Autodesk Inventor part; units mm, degrees
ref_plane "YZ Plane" through (0, 0, 0) normal (1, 0, 0) x (0, 1, 0)
ref_plane "XZ Plane" through (0, 0, 0) normal (0, 1, 0) x (-1, 0, 0)
ref_plane "XY Plane" through (0, 0, 0) normal (0, 0, 1) x (1, 0, 0)
sketch "Sketch1" plane through (0, 0, 0) normal (0, 1, 0) x (-1, 0, 0)
  line L0 (0, 0) -> (90, 0)
  line L1 (90, 0) -> (90, -45)
  line L2 (90, -45) -> (0, -45)
  line L3 (0, -45) -> (0, 0)
  dimension "d0" = 90
  dimension "d1" = 45
extrude "Extrusion1" add sketch "Sketch1" along normal blind 45
sketch "Sketch2" plane through (0, 45, 0) normal (0, 1, 0) x (1, 0, 0)
  point P0 (0, 0)
shell "Shell1" thickness 1.5 removed faces 1 at (-30, 45, -15)
sketch "Sketch3" plane through (-90, 0, 0) normal (0, 0, 1) x (1, 0, 0)
  line L0 (75, 35) -> (65, 35)
  line L1 (1.5, 45) -> (88.5, 45)
  line L2 (75, 35) -> (65, 35)
  line L3 (65, 35) -> (65, 45)
  line L4 (65, 45) -> (75, 45)
  line L5 (75, 45) -> (75, 35)
  point P0 (90, 0)
extrude "Extrusion2" cut sketch "Sketch3" against normal blind 10
sketch "Sketch4" plane through (0, 0, -45) normal (0, 0, -1) x (-1, 0, 0)
  line L0 (45, 45) -> (53.3446, 45)
  line L1 (53.3446, 45) -> (53.3446, 39.0799)
  line L2 (53.3446, 39.0799) -> (45, 39.0799)
  line L3 (45, 39.0799) -> (45, 45)
  point P0 (0, 0)
extrude "Extrusion3" cut sketch "Sketch4" against normal blind 10
properties part number "Scannerboxbottom"
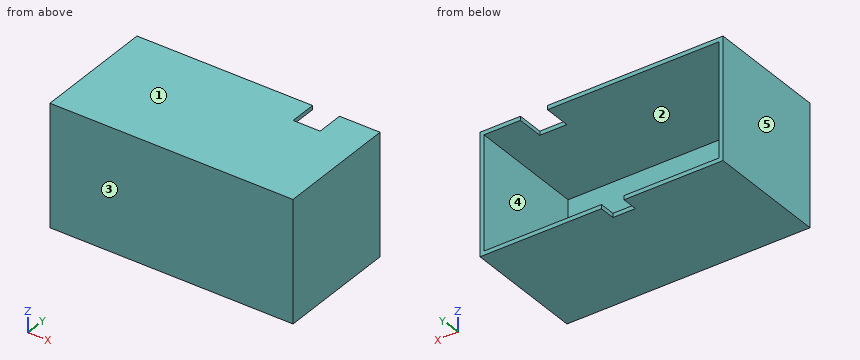
Design review of the part built by this model. Coordinates are the model's own, in mm. Face numbers are marked on the shaded views. A direction names the side the tool comes from. Coordinates: 2 decimals unless noted, no trailing zeros. Loops run counter-clockwise (first coordinate to the right, second up) from the corner with the lowest first, then second, coordinate; pieces in that order, holes last. Notation, with made-up numbers: (-25.5, 18) -> (-11.5, 18) arc R19 ccw to (-11.5, 47) -> close; hole circle Ø11 at (83, 33.25). An arc over 180 degrees is marked (long way). Answer as a JSON object with one key per item and string values.
Q1. Take a section at C-C on x = -36.5. Give the boundary of the cut face in (y, z).
Answer block:
{"outline": "(0, -45) -> (45, -45) -> (45, -43.5) -> (1.5, -43.5) -> (1.5, -1.5) -> (45, -1.5) -> (45, 0) -> (0, 0) -> close"}
Q2. The part is to be moulded in two halves that separate along Z. For the marked faces 1, 2 and 3, say which applies: +Z half, -Z half, draft (parallel to the pull), parting line (faces both ways), or undercut.
Answer block:
{"face 1": "+Z half", "face 2": "undercut", "face 3": "draft"}
Q3. Take a section at A-A on y = 13.5. Give the boundary of the cut face in (x, z), plus the area to 3 significant figures.
Answer block:
{"outline": "(-90, -45) -> (0, -45) -> (0, 0) -> (-90, 0) -> close; hole (-88.5, -43.5) -> (-1.5, -43.5) -> (-1.5, -1.5) -> (-88.5, -1.5) -> close", "area": "396 mm^2"}
Q4. Take a section at B-B on z = -19. Give the boundary of the cut face in (x, y).
Answer block:
{"outline": "(-90, 0) -> (0, 0) -> (0, 45) -> (-1.5, 45) -> (-1.5, 1.5) -> (-88.5, 1.5) -> (-88.5, 45) -> (-90, 45) -> close"}
Q5. To check wall thickness, follow L1, parallel to X at y = 14, z = -7.5; L2, parallel to Z at x = -21, y = 4; L3, parallel to Y at x = -38, z = -6. State the ranges of each line that lie inside material, in increasing order.
Answer block:
{"L1": "x = -90 to -88.5, -1.5 to 0", "L2": "z = -45 to -43.5, -1.5 to 0", "L3": "y = 0 to 1.5"}
Q6. Clearance check with flat-ended pins moving along their axes: pin 1 Ø0.8 at (x, z) = (-18, -0.5) entering from +Y; pin 2 Ø1.2 at (x, z) = (-50, -44) entering from +Y; pin 3 Ø3 at (x, z) = (-24.5, -6) entering from +Y. State where each tip first meets the part, or that it passes through.
Answer block:
{"pin 1": "stops at y = 35", "pin 2": "stops at y = 39.08", "pin 3": "stops at y = 1.5"}
Q7. Tool access review of the marked faces 4 and 5: name each direction out of +Z, -Z, +X, -X, +Y, -Y from which nothing blocks a thin tool from reaching the whole face with its end or side.
Answer block:
{"face 4": "+Y", "face 5": "+Z, -Z, -X, +Y, -Y"}
